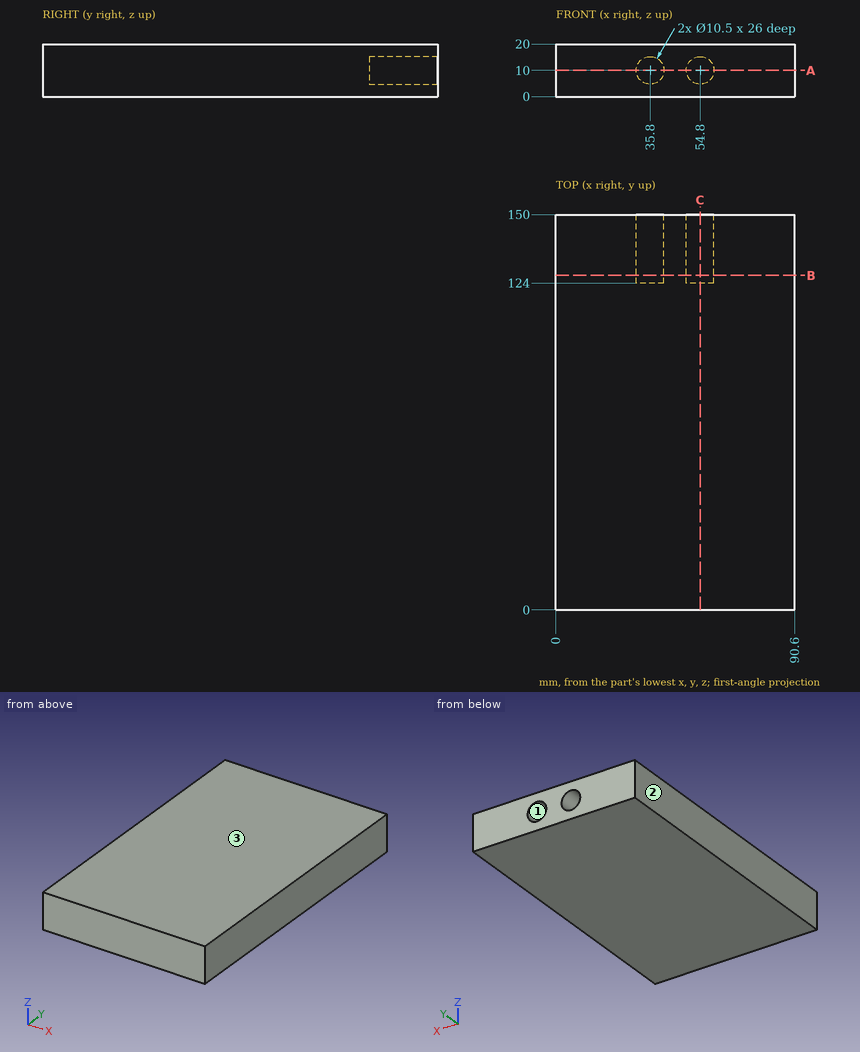
Study the drawing (mm; zero at the part's minimum x, y, z) and answer. Coordinates: 2 decimals unless noted, no trailing zeros. Loops run counter-clockwise (first coordinate to the right, second up) from the corner with the lowest first, then second, coordinate; pieces in that order, holes last. Notation, with made-up numbers: M 72,-17.75 L 100,-17.75 A21 cw 100,18.25 Z; hole C 8.25,2.5 d9. An arc over 180 degrees is marked long. Answer in a Markdown table with one row per item. Add a question column.
1. Find section B-B, the plane y = 127. Write down the section's boundary in (x, z).
2. Consider L1, parallel to X at y = 139.25, z = 10; L2, parallel to X at y = 137.5, z = 6.75; L3, parallel to Z at x = 56.5, y = 139. Determine where each line is inside the solid, lowest interval first.
3. Find section C-C, the plane x = 54.8. Write down the section's boundary in (y, z), then the cut area to 3 significant figures.
4. The mould has two halves that part along X. Classify the marked faces 1, 2 and 3: pulls with the +X half, pulls with the -X half, needs draft (parallel to the pull), parting line crosses it, or undercut.
5. Find section A-A, the plane z = 10. Write down the section's boundary in (x, y), then the cut area to 3 significant figures.
6. A flat-ended cylindrical pin translates along its axis: P1, Ø3, axis at x = 57, z = 8, coming from the +Y side. Find the tip coordinate at first contact, or state that the pin passes through.
Reported:
| question | item | result |
|---|---|---|
| 1 | outline | M 0,0 L 90.6,0 L 90.6,20 L 0,20 Z; hole C 35.8,10 d10.5; hole C 54.8,10 d10.5 |
| 2 | L1 | x = 0 to 30.55, 41.05 to 49.55, 60.05 to 90.6 |
| 2 | L2 | x = 0 to 31.68, 39.92 to 50.68, 58.92 to 90.6 |
| 2 | L3 | z = 0 to 5.03, 14.97 to 20 |
| 3 | outline | M 0,0 L 150,0 L 150,4.75 L 124,4.75 L 124,15.25 L 150,15.25 L 150,20 L 0,20 Z |
| 3 | area | 2,730 mm^2 |
| 4 | face 1 | undercut |
| 4 | face 2 | pulls with the -X half |
| 4 | face 3 | needs draft |
| 5 | outline | M 0,0 L 90.6,0 L 90.6,150 L 60.05,150 L 60.05,124 L 49.55,124 L 49.55,150 L 41.05,150 L 41.05,124 L 30.55,124 L 30.55,150 L 0,150 Z |
| 5 | area | 13,000 mm^2 |
| 6 | P1 | stops at y = 124 |
